Autodesk Inventor part; units mm, degrees
ref_plane "YZ Plane" through (0, 0, 0) normal (1, 0, 0) x (0, 1, 0)
ref_plane "XZ Plane" through (0, 0, 0) normal (0, 1, 0) x (-1, 0, 0)
ref_plane "XY Plane" through (0, 0, 0) normal (0, 0, 1) x (1, 0, 0)
sketch "Sketch1" plane through (0, 0, 0) normal (0, 0, 1) x (1, 0, 0)
  line L0 (0, 0) -> (609.6, 0)
  line L1 (609.6, 0) -> (609.6, 304.8)
  line L2 (609.6, 304.8) -> (0, 304.8)
  line L3 (0, 304.8) -> (0, 0)
  dimension "d0" = 609.6
  dimension "d1" = 304.8
extrude "Extrusion1" add sketch "Sketch1" along normal blind 152.4
sketch "Sketch2" plane through (0, 0, 152.4) normal (0, 0, 1) x (1, 0, 0)
  line L0 (0, 0) -> (0, 304.8)
  line L1 (609.6, 0) -> (0, 0)
  line L2 (609.6, 304.8) -> (609.6, 0)
  line L3 (0, 304.8) -> (609.6, 304.8)
  line L4 (6.35, 6.35) -> (603.25, 6.35)
  line L5 (603.25, 6.35) -> (603.25, 298.45)
  line L6 (603.25, 298.45) -> (6.35, 298.45)
  line L7 (6.35, 298.45) -> (6.35, 6.35)
  dimension "d4" = 6.35
  dimension "d5" = 6.35
  dimension "d6" = 6.35
  dimension "d7" = 6.35
extrude "Extrusion2" cut sketch "Sketch2" against normal blind 146.05 contours L7 L6 L5 L4
properties part number "electrical shelfing" material "Aluminum-6061"
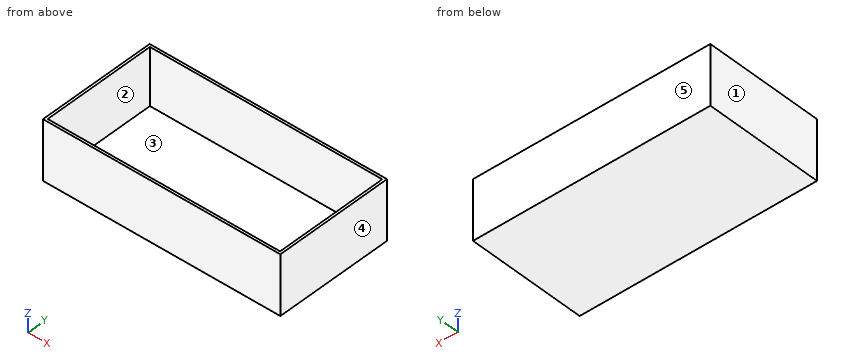
For this review, take the finished solid that the model builds, in its own axes (mm). Face numbers are marked on the shaded views. A direction names the side the tool comes from. Coordinates: 2 decimals unless noted, no trailing zeros. Loops run counter-clockwise (first coordinate to the right, second up) from the corner with the lowest first, then second, coordinate; pieces in that order, holes last. Notation, with made-up numbers: (2, -21) - (48, -21) arc R29 cw to (48, 17) - close; hole circle Ø5 at (40, 35). An arc over 180 degrees is marked (long way). Return JSON: item names as keys, results as strings.
Item 1: For line 1 (Y direction, x = 285, z = 99.5); line 2 (X direction, y = 59, z = 92.5); line 3 (Z direction, x = 336.5, y = 205.5), list the stretches that pass through material, from the lowest coordinate up.
Determined:
{"line 1": "y = 0 to 6.35, 298.45 to 304.8", "line 2": "x = 0 to 6.35, 603.25 to 609.6", "line 3": "z = 0 to 6.35"}
Item 2: Take a section at C-C (x = 557). Give the boundary of the cut face in (y, z).
Determined:
{"outline": "(0, 0) - (304.8, 0) - (304.8, 152.4) - (298.45, 152.4) - (298.45, 6.35) - (6.35, 6.35) - (6.35, 152.4) - (0, 152.4) - close"}
Item 3: Take a section at B-B (y = 233). Give the boundary of the cut face in (x, z).
Determined:
{"outline": "(0, 0) - (609.6, 0) - (609.6, 152.4) - (603.25, 152.4) - (603.25, 6.35) - (6.35, 6.35) - (6.35, 152.4) - (0, 152.4) - close"}
Item 4: Take a section at A-A (z = 134). Give the boundary of the cut face in (x, y).
Determined:
{"outline": "(0, 0) - (609.6, 0) - (609.6, 304.8) - (0, 304.8) - close; hole (6.35, 6.35) - (603.25, 6.35) - (603.25, 298.45) - (6.35, 298.45) - close"}
Item 5: Insertion check: pin 1 (5 mm diameter, centred on x = 445, y = 195, fed in from +Z). The pin has a flat end and moves straight along its axis. Give the tip position at first contact, or say it passes through.
Determined:
{"pin 1": "stops at z = 6.35"}
Item 6: For the marked faces 1 and 2, list the 3-axis set-ups (+Z, -Z, +X, -X, +Y, -Y) from which the entire face can be reached by the end or side of a thin tool; tool diameter is ignored.
Determined:
{"face 1": "+Z, -Z, -X, +Y, -Y", "face 2": "+Z"}
Item 7: Mouldability with a two-part tool opening along X and no side actions: class the marked faces 3, 4 and 5 as pulls with the +X half, pulls with the -X half, needs draft (parallel to the pull), parting line crosses it, or undercut.
Determined:
{"face 3": "undercut", "face 4": "pulls with the +X half", "face 5": "needs draft"}
